Could you check a few things on this model? Use its own coordinates, in mm. Give positions to 0.01 mm unless a question says otherwise; leave off trailing zeros. Loops run counter-clockwise (first coordinate to the right, second up) from the corner with the lowest first, then second, coordinate; pieces in that order, holes last. Notation, with made-up numbers: (79, -23.5) - (120, -23.5) arc R20 ccw to (120, 15.5) - close; hole circle Ø5 at (-15.75, 45). An arc over 180 degrees is marked (long way). Answer in a Markdown table with one row per item. Add a question column.
Autodesk Inventor part; units mm, degrees
ref_plane "WorkPlane2" through (0, 0, 0) normal (0, 0, 1) x (1, 0, 0)
ref_plane "Work Plane2" through (0, 0, -3.7) normal (0, 0, 1) x (1, 0, 0)
ref_plane "WorkPlane3" through (0, 0, 7) normal (0, 0, 1) x (1, 0, 0)
ref_plane "WorkPlane2" through (0, 0, 0) normal (0, 0, 1) x (1, 0, 0)
sketch "Sketch1" plane through (0, 0, 0) normal (1, 0, 0) x (0, 1, 0)
  point P0 (0, 0)
ref_plane "Work Plane2" through (0, 0, -3.7) normal (0, 0, 1) x (1, 0, 0)
ref_plane "WorkPlane3" through (0, 0, 7) normal (0, 0, 1) x (1, 0, 0)
sketch "Sketch2" plane through (0, 0, 0) normal (0, 1, 0) x (-1, 0, 0)
  point P0 (0, 0)
sketch "Sketch3" plane through (0, 0, 0) normal (1, 0, 0) x (0, 1, 0)
  line L0 (2, -5.1) -> (1.65, -4.4)
  line L1 (2, -26) -> (2, -5.1)
  line L2 (0, -26) -> (2, -26)
  line L3 (0, 0) -> (0, -26)
  arc A0 (4.2, -1) -> (0, 0) centre (0, -9.32) ccw
  line L4 (4.2, -1.15) -> (4.2, -1)
  line L5 (1.65, -3.7) -> (4.2, -1.15)
  line L6 (1.65, -4.4) -> (1.65, -3.7)
  line L7 (0, -31.6445) -> (0, 31.6445) construction
  line L8 (0, -31.6445) -> (0, 31.6445)
  line L9 (0, -44.3023) -> (0, 44.3023)
  dimension "d2" = 2
  dimension "d4" = 1.65
  dimension "d6" = 0.7
  dimension "d8" = 2.7
  dimension "d10" = 135
  dimension "d12" = 4.2
  dimension "d14" = 0
  dimension "d16" = 1
  dimension "d18" = 25
  dimension "d22" = 20.9
revolve "Revolution1" add sketch "Sketch3" angle 360 about axis through (0, 0, -31.6445) along (0, 0, 1)
fillet "Fillet1" radius 1 1 edges at (0, -1.65, -3.7)
sketch "Sketch4" plane through (0, 0, 0) normal (0, 1, 0) x (-1, 0, 0)
  line L0 (0, 0) -> (-2.6, 0)
  line L1 (0, -2.1667) -> (0, 0)
  line L2 (-2.6, 0) -> (-0.4333, -2.1667)
  line L3 (0, -11.184) -> (0, 1.864)
  arc A0 (4.2, -1) -> (-4.2, -1) centre (0, -9.32) ccw
  line L4 (0, -2.1667) -> (-0.4333, -2.1667)
  point P0 (0, -2.6)
  dimension "d30" = 45
  dimension "d33" = 5.2
  dimension "d34" = 0.4333
  dimension "d35" = 90
extrude "Extrusion1" cut sketch "Sketch4" along normal mid plane 0.8667
pattern_circular "PolarArray1" count 4 over 360 about axis through (0, 0, -10) along (0, 0, 1) of "Extrusion1"
thread "Thread1"
ref_plane "MSC_PF1" through (0, 0, 0) normal (1, 0, 0) x (0, 1, 0)
ref_plane "MSC_PT1" through (0, 4.2, -1.15) normal (0, 0, -1) x (-1, 0, 0)
equation "\"d2\" = 0.5 * NND"
equation "\"d4\" = 0.5 * msp_mdtds"
equation "\"d6\" = msp_x"
equation "\"d8\" = ParK"
equation "\"d12\" = 0.5 * Dk"
equation "\"d16\" = ParF"
equation "\"d18\" = NLG"
equation "\"d22\" = b"
equation "\"d24\" = r"
equation "\"d33\" = M"
equation "\"d31\" = 0.166667 * M"
equation "\"d39\" = b"
equation "\"PTC\" = 0.7"
equation "\"msp_x\" = PTC"
equation "\"NLG\" = 25"
equation "\"NND\" = 4"
equation "\"ParK\" = 2.7"
equation "\"r\" = 1"
equation "\"msp_mdtds\" = NND - PTC"
equation "\"b\" = 20.9"
equation "\"Dk\" = 8.4"
equation "\"ParF\" = 1"
equation "\"M\" = 5.2"
equation "\"ParA\" = 1.4"
equation "\"THREADDIA\" = NND"
equation "\"TEMPLATE\" = 1.2345"
properties part number "ISO 7047 - M4x25 - 4.8 - H" material "Steel"
(1) We'd pull the mould along X, two halves only. Please class faces 1 (the flat face through (0, 0, -26)), 2 (the flat face through (0, 1.4, -1.2)), 3 (the conical face through (2.03, -0.45, -3.27)), 4 (the flat face through (0.433, 1, -1)): pulls with the +X half, pulls with the -X half, needs draft (parallel to the pull), parting line crosses it, or undercut.
(2) Please list where these lines run through material, in increasing order: line 1 (Z direction, x = -1, y = -1.5); line 2 (X direction, y = -0.5, z = -24.5); line 3 (Y direction, x = 2, z = -2.75).
(3) I want a section at A-A on z = -16.5. Please give me the cut outline in (x, y), then the cut area to 3 significant figures.
(4) For pin 1 Ø0.9 at (y, z) = (-1.5, -1.5) entering from +X; pin 2 Ø0.9 at (y, z) = (1, -1.5) entering from +X; pin 3 Ø2 at (x, y) = (-3, -3.5) entering from +Z, each with a flat end and sliding along its axis, tell me the tip position at first contact or that it passes through.
Reported:
| question | item | result |
|---|---|---|
| 1 | face 1 | needs draft |
| 1 | face 2 | undercut |
| 1 | face 3 | parting line crosses it |
| 1 | face 4 | undercut |
| 2 | line 1 | -26 to -4.71, -3.58 to -0.18 |
| 2 | line 2 | -1.94 to 1.94 |
| 2 | line 3 | -1.66 to 1.66 |
| 3 | outline | circle Ø4 at (0, 0) |
| 3 | area | 12.6 mm² |
| 4 | pin 1 | x = 4.02 |
| 4 | pin 2 | x = 4.14 |
| 4 | pin 3 | z = -0.73 |
